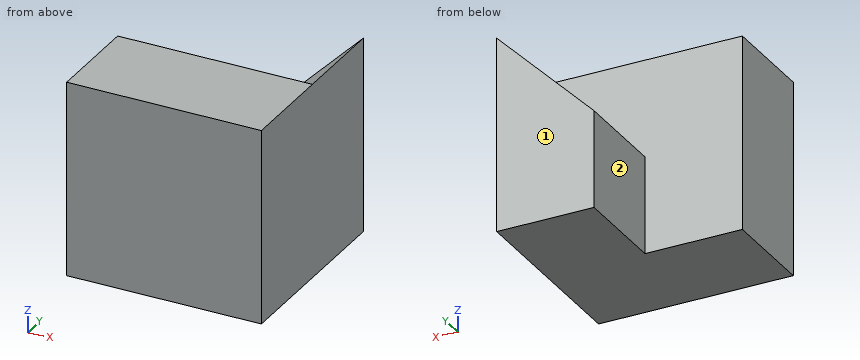
from build123d import *

# Parameters (mm, degrees)
SKETCH1_W           = 40
SKETCH1_H           = 20
BOSS_EXTRUDE1_DEPTH = 40
SKETCH2_W           = 20
SKETCH2_H           = 20
BOSS_EXTRUDE2_DEPTH = 40
CUT_EXTRUDE2_DEPTH  = 20
CUT_EXTRUDE3_DEPTH  = 20
BOSS_EXTRUDE3_DEPTH = 20
BOSS_EXTRUDE4_DEPTH = 20
CUT_EXTRUDE4_DEPTH  = 20


with BuildPart() as part:
    # Sketch1 → Boss-Extrude1 (new body)
    with BuildSketch(Plane.XY):
        with Locations((20, 10)):
            Rectangle(SKETCH1_W, SKETCH1_H)
    extrude(amount=BOSS_EXTRUDE1_DEPTH)

    # Sketch2 → Boss-Extrude2 (add)
    with BuildSketch(Plane.XY.offset(40)):
        with Locations((30, 30)):
            Rectangle(SKETCH2_W, SKETCH2_H)
    extrude(amount=-BOSS_EXTRUDE2_DEPTH)

    # Sketch3 → Cut-Extrude2 (cut)
    with BuildSketch(Plane(origin=(0, 40, 0), x_dir=(1, 0, 0), z_dir=(0, 1, 0))):
        Polygon((40, -40), (40, -20), (20, -40), align=None)
    extrude(amount=-CUT_EXTRUDE2_DEPTH, mode=Mode.SUBTRACT)

    # Sketch4 → Cut-Extrude3 (cut)
    with BuildSketch(Plane(origin=(0, 40, 0), x_dir=(1, 0, 0), z_dir=(0, 1, 0))):
        Polygon((40, 0), (20, -20), (20, 0), align=None)
    extrude(amount=-CUT_EXTRUDE3_DEPTH, mode=Mode.SUBTRACT)

    # Sketch5 → Boss-Extrude3 (add)
    with BuildSketch(Plane(origin=(0, 20, 0), x_dir=(1, 0, 0), z_dir=(0, 1, 0))):
        Polygon((20, 0), (20, -20), (40, 0), align=None)
    extrude(amount=BOSS_EXTRUDE3_DEPTH)

    # Sketch6 → Boss-Extrude4 (add)
    with BuildSketch(Plane(origin=(0, 20, 0), x_dir=(1, 0, 0), z_dir=(0, 1, 0))):
        Polygon((20, -40), (40, -40), (40, -20), align=None)
    extrude(amount=BOSS_EXTRUDE4_DEPTH)

    # Sketch7 → Cut-Extrude4 (cut)
    with BuildSketch(Plane(origin=(0, 40, 0), x_dir=(1, 0, 0), z_dir=(0, 1, 0))):
        Polygon((20, -20), (20, -40), (30, -30), align=None)
        Polygon((30, -30), (20, -40), (40, -40), align=None)
    extrude(amount=-CUT_EXTRUDE4_DEPTH, mode=Mode.SUBTRACT)


solid = part.part
The listing builds one solid part. Answer for the finished solid, in the listing's coordinates (mm). Face numbers are marked on the shaded views. A direction names the side the tool comes from. Give positions to 0.01 mm unless a question says otherwise; leave off trailing zeros. Write each loop counter-clockwise with the first axis right and the second up, starting at its lowest first coordinate (ties: lowest second). Pieces come first, ordered by that corner, then holes. Notation, with made-up numbers: (45.5, 35) -> (88.5, 35) arc R13 cw to (88.5, 60) -> close; hole circle Ø1 at (17.25, 73). An arc over 180 degrees is marked (long way). Use a Markdown table: item, result.
(1) Section B-B, the plane x = 32.5 is taken. Determine the outline of the cut face in (y, z), then the cut area to 3 significant figures.
Return value:
| item | result |
|---|---|
| outline | (0, 0) -> (40, 0) -> (40, 32.5) -> (20, 32.5) -> (20, 40) -> (0, 40) -> close |
| area | 1,450 mm2 |
(2) For the marked faces 1 and 2, determine the directions among +Z, -Z, +X, -X, +Y, -Y from which every point of the face is accessible in a straight line to the end or side of a thin tool.
Return value:
| item | result |
|---|---|
| face 1 | +Z, -Z, +X, -X, +Y |
| face 2 | +Z, -Z, -X, +Y |
(3) Section C-C, the plane y = 33 is taken. Determine the outline of the cut face in (x, z).
Return value:
| item | result |
|---|---|
| outline | (20, 0) -> (40, 0) -> (40, 40) -> (20, 20) -> close |
(4) Flat-ended cylindrical pins translate along their axes: P1, Ø16, axis at y = 31, z = 11, coming from the -X side; P2, Ø4, axis at y = 30, z = 31.5, coming from the -X side. Find the tip coordinate at first contact, or state that the pin passes through.
Return value:
| item | result |
|---|---|
| P1 | x = 20 |
| P2 | x = 29.5 |
(5) Find the intervals of material crossed by probe 1 along Y at (x, z) = (7.5, 34.5); probe 2 along X at (y, z) = (38, 2.5); probe 3 along Z at (x, y) = (30, 29.5), in increasing order. Write a range as from..to.
Return value:
| item | result |
|---|---|
| probe 1 | 0..20 |
| probe 2 | 20..40 |
| probe 3 | 0..30 |
(6) Section A-A, the plane z = 35 is taken. Determine the outline of the cut face in (x, y).
Return value:
| item | result |
|---|---|
| outline | (0, 0) -> (40, 0) -> (40, 40) -> (35, 40) -> (35, 20) -> (0, 20) -> close |
(7) Section D-D, the plane x = 17 is taken. Determine the outline of the cut face in (y, z).
Return value:
| item | result |
|---|---|
| outline | (0, 0) -> (20, 0) -> (20, 40) -> (0, 40) -> close |
